Can you work these out from the model? Positions are in its coordinate system, mm. Round coordinates to 2 decimals unless told otherwise and drop trailing zeros. Loops run counter-clockwise (first coordinate to the right, second up) from the corner with the lowest first, then second, coordinate; pieces in that order, holes last.
from build123d import *

# Parameters (mm, degrees)
F0_W     = 882.65
F0_H     = 209.55
F0_W_2   = 57.15
F0_H_2   = 79.375
F0_W_3   = 107.95
F0_H_3   = 146.05
F1_DEPTH = 3.175


with BuildPart() as f1:
    # F0 (on Top) → F1 (new body, symmetric)
    with BuildSketch(Plane.XY):
        Rectangle(F0_W, F0_H)
        with Locations((-346.075, 4.7625)):
            Rectangle(F0_W_2, F0_H_2, mode=Mode.SUBTRACT)
        with Locations((0, 4.7625)):
            Rectangle(F0_W_3, F0_H_3, mode=Mode.SUBTRACT)
        with Locations((346.075, 4.7625)):
            Rectangle(F0_W_2, F0_H_2, mode=Mode.SUBTRACT)
    extrude(amount=F1_DEPTH, both=True)


solid = f1.part
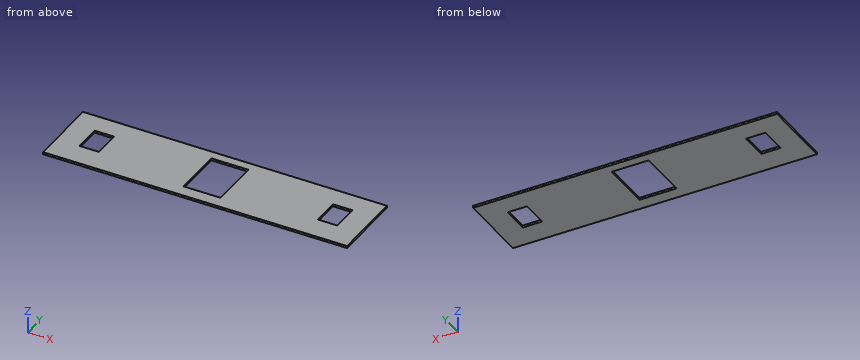
(1) If I drill on line 1 (X direction, y = 25, z = -0.75) (3 decimals); line 2 (X direction, y = -40, z = -2.75) (3 decimals); line 3 (Y direction, x = -2, z = -3) (1 decimal), over which ranges is the centre line in solid material (lowest first)?
Worked answers:
line 1: x = -441.325 to -374.65, -317.5 to -53.975, 53.975 to 317.5, 374.65 to 441.325
line 2: x = -441.325 to -53.975, 53.975 to 441.325
line 3: y = -104.8 to -68.3, 77.8 to 104.8
(2) If we section it at B-B, the plane z = -2: State how many separate pieces and enclosed holes the cut face has, then the cut area to 3 significant figures.
Worked answers:
separate pieces: 1
enclosed holes: 3
area: 160,000 mm2
(3) If we section it at D-D, the plane x = 348.5: List the corners of the cut face in (y, z) for me (3 decimals).
Worked answers:
outline: (-104.775, -3.175) - (-34.925, -3.175) - (-34.925, 3.175) - (-104.775, 3.175) - close; (44.45, -3.175) - (104.775, -3.175) - (104.775, 3.175) - (44.45, 3.175) - close
(4) If we section it at A-A, the plane y = 14.5: List the corners of the cut face in (x, z) for me (3 decimals).
Worked answers:
outline: (-441.325, -3.175) - (-374.65, -3.175) - (-374.65, 3.175) - (-441.325, 3.175) - close; (-317.5, -3.175) - (-53.975, -3.175) - (-53.975, 3.175) - (-317.5, 3.175) - close; (53.975, -3.175) - (317.5, -3.175) - (317.5, 3.175) - (53.975, 3.175) - close; (374.65, -3.175) - (441.325, -3.175) - (441.325, 3.175) - (374.65, 3.175) - close
(5) If we section it at C-C, the plane y = -54.5: List the corners of the cut face in (x, z) for me (3 decimals).
Worked answers:
outline: (-441.325, -3.175) - (-53.975, -3.175) - (-53.975, 3.175) - (-441.325, 3.175) - close; (53.975, -3.175) - (441.325, -3.175) - (441.325, 3.175) - (53.975, 3.175) - close
